Verification items for the finished model (mm, model axes). A direction names the side the tool comes from. Give positions to 0.01 mm unless a question says otherwise; leave off trailing zeros. Loops run counter-clockwise (first coordinate to the right, second up) from the corner with the lowest first, then second, coordinate; pieces in that order, holes last. Notation, with made-up numbers: (75, 22.25) - (79, 22.25) arc R23 cw to (79, 56.25) - close; hole circle Ø2 at (-39, 60). An arc over 180 degrees is marked (long way). Use one line per item in the form item = value.
```python
from build123d import *

# Parameters (mm, degrees)
SKETCH1_W           = 25.4
SKETCH1_H           = 25.4
SKETCH1_W_2         = 19.05
SKETCH1_H_2         = 19.05
BOSS_EXTRUDE1_DEPTH = 279.4
SKETCH7_R           = 1.905
CUT_EXTRUDE1_DEPTH  = 281.839473721
SKETCH8_R           = 1.905
SKETCH8_R_2         = 6.35
CUT_EXTRUDE2_DEPTH  = 281.839473721


with BuildPart() as part:
    # Sketch1 → Boss-Extrude1 (new, symmetric)
    with BuildSketch(Plane.XY):
        Rectangle(SKETCH1_W, SKETCH1_H)
        Rectangle(SKETCH1_W_2, SKETCH1_H_2, mode=Mode.SUBTRACT)
    extrude(amount=BOSS_EXTRUDE1_DEPTH, both=True)

    # Sketch7 → Cut-Extrude1 (cut, through all)
    with BuildSketch(Plane(origin=(0, 12.7, 0), x_dir=(1, 0, 0), z_dir=(0, 1, 0))):
        with Locations(Location((0, -266.7, 0), (0, 0, 270))):
            Circle(SKETCH7_R)
    extrude(amount=-CUT_EXTRUDE1_DEPTH, mode=Mode.SUBTRACT)

    # Sketch8 → Cut-Extrude2 (cut, through all)
    with BuildSketch(Plane(origin=(12.7, 0, 0), x_dir=(0, 0, -1), z_dir=(1, 0, 0))):
        with Locations(Location((215.9, 0, 0), (0, 0, 90))):
            Circle(SKETCH8_R)
        with Locations(Location((263.652, 0, 0), (0, 0, 90))):
            Circle(SKETCH8_R)
        with Locations(Location((239.7125, 0, 0), (0, 0, 90))):
            Circle(SKETCH8_R_2)
    extrude(amount=-CUT_EXTRUDE2_DEPTH, mode=Mode.SUBTRACT)


solid = part.part
```
1. Draft check along Y on faces 3 (the flat face through (0, -9.525, 4)), 4 (the flat face through (11, 0, 279.4)), 5 (the flat face through (0, 12.7, 4)). Enter one of: released by +Y, released by -Y, zero draft, split by the parting line, or undercut.
Result set:
face_3 = undercut
face_4 = zero draft
face_5 = released by +Y
2. Tool access check on faces 1 (the flat face through (9.525, 0, 4)), 2 (the flat face through (-12.7, 0, 4)). Record the directions out of +Z, -Z, +X, -X, +Y, -Y that give a thin tool (end or side, any length) a straight path to the whole face; none if there is none.
Result set:
face_1 = +Z, -Z
face_2 = +Z, -Z, -X, +Y, -Y
3. Depth check by flat-ended pin: pin 1 Ø2 at (x, y) = (6.5, 7) entering from +Z; pin 2 Ø5 at (y, z) = (0, -263.652) entering from +X. Enter the tip coordinate at first touch or a pass-through.
Result set:
pin_1 = through
pin_2 = 12.7
4. Scan lines: probe 1 along Z at (x, y) = (12, 0) (1 decimal); probe 2 along Y at (x, z) = (-2.5, -159.5) (3 decimals). Record each from-to range of solid material in increasing order.
Result set:
probe_1 = -279.4 to -265.6, -261.7 to -246.1, -233.4 to -217.8, -214 to 279.4
probe_2 = -12.7 to -9.525, 9.525 to 12.7
5. Section check A-A, the plane z = 180.5. Record the cut outline in (x, y) (3 decimals), then the cut area to 3 significant figures.
Result set:
outline = (-12.7, -12.7) - (12.7, -12.7) - (12.7, 12.7) - (-12.7, 12.7) - close; hole (-9.525, -9.525) - (9.525, -9.525) - (9.525, 9.525) - (-9.525, 9.525) - close
area = 282 mm²
